Can you work these out from the drawing? Everything is in mm from the part's minimum corner. A direction names the side the tool comes from. Round coordinates to 2 decimals unless told otherwise and drop trailing zeros. Order: outer loops, then holes, each group sorted by start corner. A loop starts at its lowest first (then second) coordinate and runs counter-clockwise, first axis right, second up. Notation, with made-up numbers: (-40, 44.5) - (-36, 44.5) arc R13 ccw to (-36, 62.5) - close; hole circle Ø3 at (-29, 8.25). An arc over 180 degrees is marked (long way). Write item = value, one per line.
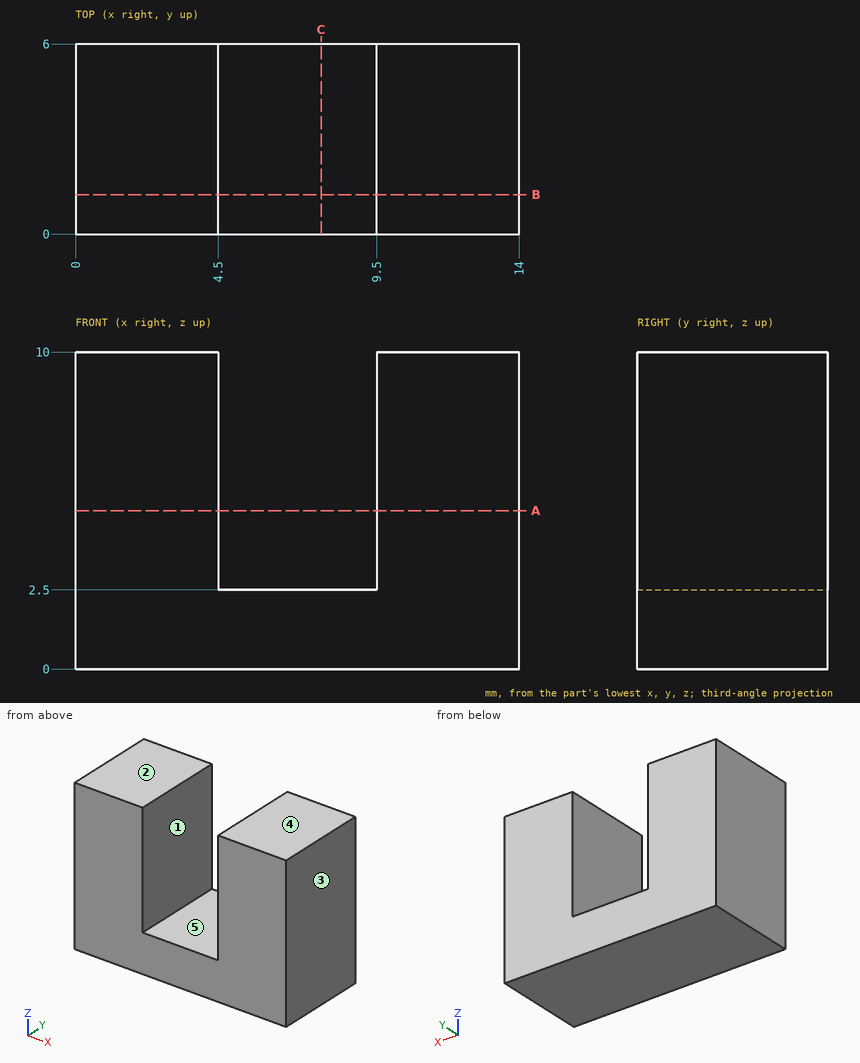
(1) If we section it at A-A (z = 5): Write out the boundary of the cut face in (x, y).
Computed:
outline = (0, 0) - (4.5, 0) - (4.5, 6) - (0, 6) - close; (9.5, 0) - (14, 0) - (14, 6) - (9.5, 6) - close
(2) Will these pins go through, and if not, where does the flat tip stop? P1, Ø1.5, axis at x = 12, y = 1.5, coming from the -Z side; P2, Ø1.5, axis at x = 7.5, y = 2, coming from the +Z side.
Computed:
P1 = 0
P2 = 2.5
(3) Thinking about a two-plate mould opening in X: for the marked faces 1, 2 and 3, which applies, +X half, -X half, draft (parallel to the pull), parting line (faces both ways), or undercut?
Computed:
face_1 = undercut
face_2 = draft
face_3 = +X half
(4) If we section it at B-B (y = 1.25): Write out the boundary of the cut face in (x, z), plus the area to 4 significant figures.
Computed:
outline = (0, 0) - (14, 0) - (14, 10) - (9.5, 10) - (9.5, 2.5) - (4.5, 2.5) - (4.5, 10) - (0, 10) - close
area = 102.5 mm^2
(5) If I drill on line 1 (X direction, y = 4.85, z = 8.75); line 2 (Z direction, x = 6.75, y = 5.05), over which ranges is the centre line in solid material (lowest first)? Write a range as from..to.
Computed:
line_1 = 0..4.5, 9.5..14
line_2 = 0..2.5
(6) On a 3-axis mill with a long thin cutter (end or side, diameter ignored), from which of +Z, -Z, +X, -X, +Y, -Y can I reach the whole of each face in a straight line? I mean the marked faces 4 and 5. Say none if no direction works.
Computed:
face_4 = +Z, +X, -X, +Y, -Y
face_5 = +Z, +Y, -Y
(7) If we section it at C-C (x = 7.75): Write out the boundary of the cut face in (y, z).
Computed:
outline = (0, 0) - (6, 0) - (6, 2.5) - (0, 2.5) - close
